from build123d import *

# Parameters (mm, degrees)
SKETCH1_W                           = 85
SKETCH1_H                           = 42
BOTTOM_PLATE_DEPTH                  = 4
SKETCH2_R                           = 1.5
BOTTOM_PLATE_SCREW_HOLES_DEPTH      = 1
BOTTOM_PLATE_SCREW_HOLES_DEPTH_BACK = 5
SKETCH15_R                          = 1.5
TOP_PLATE_SCREWS_HOLES_DEPTH        = 1
TOP_PLATE_SCREWS_HOLES_DEPTH_BACK   = 2.5
SKETCH5_W                           = 60.4
SKETCH5_H                           = 15.7
LED_DEPTH                           = 1
LED_DEPTH_BACK                      = 5
SKETCH16_R                          = 1.75
LED_BOARD_SUPPORT_DEPTH             = 2
SKETCH17_R                          = 1
LED_BOARD_SCREWS_HOLES_DEPTH        = 5
SKETCH6_R                           = 2.15
TESTBUTTON_CUT_DEPTH                = 1
TESTBUTTON_CUT_DEPTH_BACK           = 7
SKETCH10_R                          = 3.7
TESTBUTTON_BIG_CUT_DEPTH            = 1
SKETCH13_R                          = 1.5
TEST_BOARD_SUPPORT_DEPTH            = 7
SKETCH14_R                          = 1
TEST_BOARD_SCREWS_HOLE_DEPTH        = 5
SKETCH9_R                           = 3.425
BRT_ADD_DEPTH                       = 6
SKETCH11_R                          = 1.75
POT_BOARD_SUPPORT_DEPTH             = 8
SKETCH12_R                          = 1
POT_BOARD_SCREWS_HOLE_DEPTH         = 5


with BuildPart() as part:
    # Sketch1 → Bottom Plate (new body)
    with BuildSketch(Plane.XY):
        Rectangle(SKETCH1_W, SKETCH1_H)
    extrude(amount=BOTTOM_PLATE_DEPTH)

    # Sketch2 → Bottom Plate Screw Holes (cut, two sides)
    with BuildSketch(Plane.XY.offset(4)) as bottom_plate_screw_holes_sk:
        with Locations((-39, 17.5)):
            Circle(SKETCH2_R)
        with Locations((-39, -17.5)):
            Circle(SKETCH2_R)
        with Locations((39, -17.5)):
            Circle(SKETCH2_R)
        with Locations((39, 17.5)):
            Circle(SKETCH2_R)
    extrude(amount=BOTTOM_PLATE_SCREW_HOLES_DEPTH, mode=Mode.SUBTRACT)
    extrude(bottom_plate_screw_holes_sk.sketch, amount=-BOTTOM_PLATE_SCREW_HOLES_DEPTH_BACK, mode=Mode.SUBTRACT)

    # Sketch15 → Top Plate Screws Holes (cut, two sides)
    with BuildSketch(Plane.XY.offset(4)) as top_plate_screws_holes_sk:
        with Locations((-37.5, 0)):
            Circle(SKETCH15_R)
        with Locations((37.5, 0)):
            Circle(SKETCH15_R)
    extrude(amount=TOP_PLATE_SCREWS_HOLES_DEPTH, mode=Mode.SUBTRACT)
    extrude(top_plate_screws_holes_sk.sketch, amount=-TOP_PLATE_SCREWS_HOLES_DEPTH_BACK, mode=Mode.SUBTRACT)

    # Sketch5 → LED (cut, two sides)
    with BuildSketch(Plane.XY.offset(4)) as led_sk:
        with Locations((0, 8.15)):
            Rectangle(SKETCH5_W, SKETCH5_H)
    extrude(amount=LED_DEPTH, mode=Mode.SUBTRACT)
    extrude(led_sk.sketch, amount=-LED_DEPTH_BACK, mode=Mode.SUBTRACT)

    # Sketch16 → LED Board Support (add)
    with BuildSketch(Plane(origin=(0, 0, 0), x_dir=(-1, 0, 0), z_dir=(0, 0, -1))):
        with Locations((-33.5, 17.5)):
            Circle(SKETCH16_R)
        with Locations((-10, -3)):
            Circle(SKETCH16_R)
        with Locations((33.5, -1)):
            Circle(SKETCH16_R)
        with Locations((12.5, 18.5)):
            Circle(SKETCH16_R)
        with Locations((13.75, -16.5)):
            Circle(SKETCH16_R)
    extrude(amount=LED_BOARD_SUPPORT_DEPTH)

    # Sketch17 → Led Board Screws Holes (cut)
    with BuildSketch(Plane(origin=(0, 0, -2), x_dir=(-1, 0, 0), z_dir=(0, 0, -1))):
        with Locations((-33.5, 17.5)):
            Circle(SKETCH17_R)
        with Locations((-10, -3)):
            Circle(SKETCH17_R)
        with Locations((12.5, 18.5)):
            Circle(SKETCH17_R)
        with Locations((33.5, -1)):
            Circle(SKETCH17_R)
        with Locations((13.75, -16.5)):
            Circle(SKETCH17_R)
    extrude(amount=-LED_BOARD_SCREWS_HOLES_DEPTH, mode=Mode.SUBTRACT)

    # Sketch6 → TestButton Cut (cut, two sides)
    with BuildSketch(Plane.XY.offset(4)) as testbutton_cut_sk:
        with Locations((-27.5, -11.5)):
            Circle(SKETCH6_R)
    extrude(amount=TESTBUTTON_CUT_DEPTH, mode=Mode.SUBTRACT)
    extrude(testbutton_cut_sk.sketch, amount=-TESTBUTTON_CUT_DEPTH_BACK, mode=Mode.SUBTRACT)

    # Sketch10 → TestButton Big Cut (cut)
    with BuildSketch(Plane.XY.offset(4)):
        with Locations((-27.5, -11.5)):
            Circle(SKETCH10_R)
    extrude(amount=-TESTBUTTON_BIG_CUT_DEPTH, mode=Mode.SUBTRACT)

    # Sketch13 → Test Board Support (add)
    with BuildSketch(Plane(origin=(0, 0, 0), x_dir=(-1, 0, 0), z_dir=(0, 0, -1))):
        with Locations((21.5, -7)):
            Circle(SKETCH13_R)
        with Locations((33.5, -7)):
            Circle(SKETCH13_R)
        with Locations((33.5, -16)):
            Circle(SKETCH13_R)
        with Locations((21.5, -16)):
            Circle(SKETCH13_R)
    extrude(amount=TEST_BOARD_SUPPORT_DEPTH)

    # Sketch14 → Test Board Screws Hole (cut)
    with BuildSketch(Plane(origin=(0, 0, -7), x_dir=(-1, 0, 0), z_dir=(0, 0, -1))):
        with Locations((21.5, -16)):
            Circle(SKETCH14_R)
        with Locations((21.5, -7)):
            Circle(SKETCH14_R)
        with Locations((33.5, -7)):
            Circle(SKETCH14_R)
        with Locations((33.5, -16)):
            Circle(SKETCH14_R)
    extrude(amount=-TEST_BOARD_SCREWS_HOLE_DEPTH, mode=Mode.SUBTRACT)

    # Sketch9 → Brt Add (cut)
    with BuildSketch(Plane(origin=(0, 0, 0), x_dir=(-1, 0, 0), z_dir=(0, 0, -1))):
        with Locations((-25.5, -9)):
            Circle(SKETCH9_R)
    extrude(amount=-BRT_ADD_DEPTH, mode=Mode.SUBTRACT)

    # Sketch11 → Pot Board Support (add)
    with BuildSketch(Plane(origin=(0, 0, 0), x_dir=(-1, 0, 0), z_dir=(0, 0, -1))):
        with Locations((-32.5, -4)):
            Circle(SKETCH11_R)
        with Locations((-18.5, -4)):
            Circle(SKETCH11_R)
        with Locations((-18.5, -18)):
            Circle(SKETCH11_R)
        with Locations((-32.5, -18)):
            Circle(SKETCH11_R)
    extrude(amount=POT_BOARD_SUPPORT_DEPTH)

    # Sketch12 → Pot Board Screws Hole (cut)
    with BuildSketch(Plane(origin=(0, 0, -8), x_dir=(-1, 0, 0), z_dir=(0, 0, -1))):
        with Locations((-32.5, -4)):
            Circle(SKETCH12_R)
        with Locations((-18.5, -4)):
            Circle(SKETCH12_R)
        with Locations((-18.5, -18)):
            Circle(SKETCH12_R)
        with Locations((-32.5, -18)):
            Circle(SKETCH12_R)
    extrude(amount=-POT_BOARD_SCREWS_HOLE_DEPTH, mode=Mode.SUBTRACT)


solid = part.part
Geometry check sheet. Reference: the model listing, model coordinates, mm. A direction names the side the tool comes from. Give positions to 0.01 mm unless a question says otherwise; leave off trailing zeros. Loops run counter-clockwise (first coordinate to the right, second up) from the corner with the lowest first, then second, coordinate; pieces in that order, holes last.
(1) Section check A-A on z = -4.5. Count the separate pieces of the cut face and the enclosed holes in it, then the cut area to 3 significant figures.
From the geometry:
separate pieces: 8
enclosed holes: 8
area: 41.6 mm2
(2) Section check D-D on x = 7. Record the cut outline in (y, z), then the cut area to 3 significant figures.
From the geometry:
outline: (-21, 0) - (0.3, 0) - (0.3, 4) - (-21, 4) - close; (16, 0) - (21, 0) - (21, 4) - (16, 4) - close
area: 105 mm2
(3) Section check C-C on y = 2.5. Record the cut outline in (x, z).
From the geometry:
outline: (-42.5, 0) - (-30.2, 0) - (-30.2, 4) - (-42.5, 4) - close; (30.2, 0) - (42.5, 0) - (42.5, 4) - (30.2, 4) - close
(4) Section check B-B on x = 25.5. Record the cut outline in (y, z) (3 decimals).
From the geometry:
outline: (-21, 0) - (-12.425, 0) - (-12.425, 4) - (-21, 4) - close; (-5.575, 0) - (0.3, 0) - (0.3, 4) - (-5.575, 4) - close; (16, 0) - (21, 0) - (21, 4) - (16, 4) - close
(5) Thickness scan on L1, parallel to Y at x = 39, z = 1.45; L2, parallel to Y at x = 30, z = 2.5; L3, parallel to Y at x = -12.5, z = -0.3. Record the ranges inside material, lowest first.
From the geometry:
L1: y = -21 to -19, -16 to 16, 19 to 21
L2: y = -21 to 0.3, 16 to 21
L3: y = -17.72 to -15.28, 16.75 to 17.5, 19.5 to 20.25
(6) Set-up check for faces 1 (the flat face through (-38, 0, 1.5)), 2 (the flat face through (0, 0.3, 2)), 3 (the cylindrical face through (-32.3, -7.9, -3.5)): record each of +Z, -Z, +X, -X, +Y, -Y from which the full face is reachable in a straight line by a thin tool's end or side.
From the geometry:
face 1: +Z
face 2: +Z, -Z
face 3: -Z
(7) Release check for a two-part mould opening along Y. For faces 4 (the flat face through (-21, -16, -2)), 5 (the cylindrical face through (8.383, -3.67, -0.986)), 6 (the flat face through (-12, 17, -2)) record: released by +Y, released by -Y, zero draft, split by the parting line, or undercut.
From the geometry:
face 4: undercut
face 5: split by the parting line
face 6: zero draft
(8) Depth check by flat-ended pin: pin 1 Ø1 at (x, y) = (10, -3) entering from -Z; pin 2 Ø2.5 at (x, y) = (39, 17.5) entering from -Z; pin 3 Ø0.6 at (x, y) = (19, -18) entering from -Z; pin 4 Ø1.2 at (x, y) = (-33.5, -16) entering from -Z. Enter the tip coordinate at first touch or a pass-through.
From the geometry:
pin 1: stops at z = 3
pin 2: passes through
pin 3: stops at z = -3
pin 4: stops at z = -2
